Could you check a few things on this model? Use its own coordinates, in mm. A direction names the side the tool comes from. Round coordinates to 2 decimals unless told otherwise and drop trailing zeros. Write each loop counter-clockwise with the first axis right and the second up, starting at its lowest first coordinate (ties: lowest second). Pieces come first, ordered by that corner, then holes.
```python
from build123d import *

# Parameters (mm, degrees)
SZKIC1_R                    = 3.5
DODANIE_WYCI_GNI_CIE1_DEPTH = 6
SZKIC2_R                    = 2
DODANIE_WYCI_GNI_CIE2_DEPTH = 18
SZKIC3_R                    = 1.1
WYTNIJ_WYCI_GNI_CIE1_DEPTH  = 6.5
SZKIC4_R                    = 2.3
WYTNIJ_WYCI_GNI_CIE2_DEPTH  = 3


with BuildPart() as part:
    # Szkic1 → Dodanie-wyciągnięcie1 (new body)
    with BuildSketch(Plane.XY):
        Circle(SZKIC1_R)
    extrude(amount=DODANIE_WYCI_GNI_CIE1_DEPTH)

    # Szkic2 → Dodanie-wyciągnięcie2 (add)
    with BuildSketch(Plane.XY.offset(6)):
        Circle(SZKIC2_R)
    extrude(amount=DODANIE_WYCI_GNI_CIE2_DEPTH)

    # Szkic3 → Wytnij-wyciągnięcie1 (cut, through all)
    with BuildSketch(Plane.ZY.offset(2)):
        with Locations((19.5, 0)):
            Circle(SZKIC3_R)
    extrude(amount=-WYTNIJ_WYCI_GNI_CIE1_DEPTH, mode=Mode.SUBTRACT)

    # Szkic4 → Wytnij-wyciągnięcie2 (cut)
    with BuildSketch(Plane(origin=(0, 0, 0), x_dir=(-1, 0, 0), z_dir=(0, 0, -1))):
        Circle(SZKIC4_R)
    extrude(amount=-WYTNIJ_WYCI_GNI_CIE2_DEPTH, mode=Mode.SUBTRACT)


solid = part.part
```
Q1. Imagine slicing it at A-A, the plane y = 0. Write out the boundary of the cut face in (x, z).
Q2. On a 3-axis mill with a long thin cutter (end or side, diameter ignored), from which of +Z, -Z, +X, -X, +Y, -Y can I reach the whole of each face in a straight line? I mean faces 1 (the flat face through (0, 0, 3)), 2 (the cylindrical face through (-0.028, 0.743, 18.689)), 3 (the flat face through (2, -2, 6)). Say none if no direction works.
Q3. I'm going to push flat-ended pins straight in: pin 1 Ø1.5 at (y, z) = (-1, 18.5) entering from +X; pin 2 Ø2 at (y, z) = (0, 19.5) entering from +X. Where does each tip first touch, or does it pass through?
Q4. Imagine slicing it at D-D, the plane y = 1.5. Write out the boundary of the cut face in (x, z), then the cut area to 3 significant figures.
Q5. Imagine slicing it at C-C, the plane z = 11. Write out the boundary of the cut face in (x, y).
Q6. Imagine slicing it at B-B, the plane x = 0. Write out the boundary of the cut face in (y, z), then the cut area to 3 significant figures.
Q7. If I drill on L1, parallel to Y at x = 0, z = 2.1; L2, parallel to Z at x = 0.3, y = 0; L3, parallel to Y at x = -0.5, z = 19.5, over which ranges is the centre line in solid material (lowest first)?
Q8. We'd pull the mould along X, two halves only. Please class faces 4 (the cylindrical face through (3.233, -1.341, 2.958)), 5 (the cylindrical face through (1.825, -1.4, 1.479)), 6 (the flat face through (0, 0, 24)): pulls with the +X half, pulls with the -X half, needs draft (parallel to the pull), parting line crosses it, or undercut.
Results found:
1. outline: (-3.5, 0) - (-2.3, 0) - (-2.3, 3) - (2.3, 3) - (2.3, 0) - (3.5, 0) - (3.5, 6) - (2, 6) - (2, 18.4) - (-2, 18.4) - (-2, 6) - (-3.5, 6) - close; (-2, 20.6) - (2, 20.6) - (2, 24) - (-2, 24) - close
2. face 1: -Z
2. face 2: +X, -X
2. face 3: +Z
3. pin 1: stops at x = 1.98
3. pin 2: passes through
4. outline: (-3.16, 0) - (-1.74, 0) - (-1.74, 3) - (1.74, 3) - (1.74, 0) - (3.16, 0) - (3.16, 6) - (1.32, 6) - (1.32, 24) - (-1.32, 24) - (-1.32, 6) - (-3.16, 6) - close
4. area: 75.1 mm2
5. outline: circle Ø4 at (0, 0)
6. outline: (-3.5, 0) - (-2.3, 0) - (-2.3, 3) - (2.3, 3) - (2.3, 0) - (3.5, 0) - (3.5, 6) - (2, 6) - (2, 24) - (-2, 24) - (-2, 6) - (-3.5, 6) - close; hole circle Ø2.2 at (0, 19.5)
6. area: 96.4 mm2
7. L1: y = -3.5 to -2.3, 2.3 to 3.5
7. L2: z = 3 to 18.4, 20.6 to 24
7. L3: y = -1.94 to -1.1, 1.1 to 1.94
8. face 4: parting line crosses it
8. face 5: undercut
8. face 6: needs draft
